Read the model definition and answer for the solid it produces. Units are mm, in the model's axes. Face numbers are marked on the shaded views. Round coordinates to 2 decimals unless told otherwise and drop trailing zeros. Write each loop counter-clockwise with the first axis right and the second up, starting at its lowest first coordinate (ties: lowest second). Pieces come first, ordered by that corner, then holes. Notation, with made-up numbers: (15.5, 66.5) -> (47.5, 66.5) arc R18 cw to (47.5, 99.5) -> close; hole circle Ø8 at (73, -13). An arc over 180 degrees is marked (long way). Return JSON: item names as keys, results as strings.
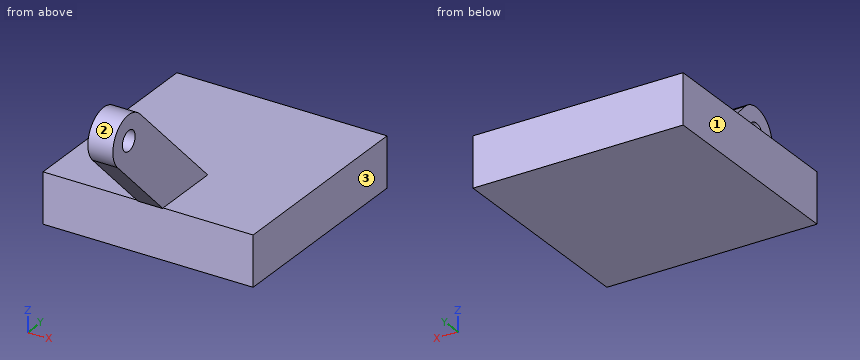
from build123d import *

# Parameters (mm, degrees)
CROQUIS1_R                    = 2
SALIENTE_EXTRUIR9_DEPTH       = 5
SALIENTE_EXTRUIR10_DEPTH      = 18
SALIENTE_EXTRUIR10_DEPTH_BACK = 24
CROQUIS7_W                    = 10
CROQUIS7_H                    = 42


with BuildPart() as part:
    # Croquis1 → Saliente-Extruir9 (new body)
    with BuildSketch(Plane(origin=(0, 0, 0), x_dir=(0, 0, -1), z_dir=(1, 0, 0))):
        with BuildLine():
            Line((0, 0), (21.213203436, 21.213203436))
            Line((21.213203436, 21.213203436), (14.142135624, 28.284271247))
            Line((14.142135624, 28.284271247), (-7.071067812, 7.071067812))
            ThreePointArc((-7.071067812, 7.071067812), (-7.071067812, 0), (0, 0))
        make_face()
        with Locations((-3.535533906, 3.535533906)):
            Circle(CROQUIS1_R, mode=Mode.SUBTRACT)
    extrude(amount=SALIENTE_EXTRUIR9_DEPTH)

    # Croquis7 → Saliente-Extruir10 (add, two sides: drawn at the far end of the back side and taken through both)
    with BuildSketch(Plane(origin=(5, 0, 0), x_dir=(0, 0, -1), z_dir=(1, 0, 0)).offset(-SALIENTE_EXTRUIR10_DEPTH_BACK)):
        with Locations((19.142135624, 35.284271247)):
            Rectangle(CROQUIS7_W, CROQUIS7_H)
    extrude(amount=SALIENTE_EXTRUIR10_DEPTH + SALIENTE_EXTRUIR10_DEPTH_BACK)


solid = part.part
Item 1: For a pull along X with two mould halves and no side action, classify the marked faces 1, 2 and 3 as released by +X, released by -X, zero draft, split by the parting line, or undercut.
Worked answers:
{"face 1": "released by -X", "face 2": "zero draft", "face 3": "released by +X"}
Item 2: Section A-A (z = 3) is taken. Give the vertices of the cut face in (x, y).
Worked answers:
{"outline": "(0, -1.44) -> (5, -1.44) -> (5, 1.61) -> (0, 1.61) -> close; (0, 5.46) -> (5, 5.46) -> (5, 11.14) -> (0, 11.14) -> close"}
Item 3: Straight lines are drawn through the part: L1, parallel to Y at x = 19, z = -23; L2, parallel to Z at x = -16, y = 47; L3, parallel to X at y = 16.5, z = -8.5. For each, find the intervals that lie inside material, in ascending order. Write a range as [from, to].
Worked answers:
{"L1": "y = [14.28, 56.28]", "L2": "z = [-24.14, -14.14]", "L3": "x = [0, 5]"}
Item 4: Section B-B (y = 16.5) is taken. Give the vertices of the cut face in (x, z), then the cut area to 3 significant figures.
Worked answers:
{"outline": "(-19, -24.14) -> (23, -24.14) -> (23, -14.14) -> (5, -14.14) -> (5, -2.36) -> (0, -2.36) -> (0, -14.14) -> (-19, -14.14) -> close", "area": "479 mm2"}
Item 5: Section D-D (x = 18) is taken. Give the vertices of the cut face in (y, z).
Worked answers:
{"outline": "(14.28, -24.14) -> (56.28, -24.14) -> (56.28, -14.14) -> (14.28, -14.14) -> close"}
Item 6: Flat-ended cylindrical pins translate along their axes: pin 1 (18.5 mm diameter, centred on y = 10.5, z = -7.5, fed in from -X); pin 2 (8 mm diameter, centred on x = 1, z = -17.5, fed in from -Y); pin 3 (8 mm diameter, centred on y = 14, z = 2.5, fed in from -X); pin 4 (1 mm diameter, centred on x = -8, y = 24, fed in from +Z). Find the tip coordinate at first contact, or state that the pin passes through.
Worked answers:
{"pin 1": "stops at x = -19", "pin 2": "stops at y = 13.5", "pin 3": "stops at x = 0", "pin 4": "stops at z = -14.14"}
Item 7: Section C-C (z = -19.5) is taken. Give the vertices of the cut face in (x, y).
Worked answers:
{"outline": "(-19, 14.28) -> (23, 14.28) -> (23, 56.28) -> (-19, 56.28) -> close"}
